Build history of the part. All positions in model axes, mm. A direction names the side the tool comes from. Coordinates: 2 decimals unless noted, no trailing zeros. Write each loop counter-clockwise with the first axis right and the second up, starting at its lowest first coordinate (ties: lowest second). Pieces come first, ordered by that corner, then holes.
Autodesk Inventor part; units mm, degrees
ref_plane "YZ Plane" through (0, 0, 0) normal (1, 0, 0) x (0, 1, 0)
ref_plane "XZ Plane" through (0, 0, 0) normal (0, 1, 0) x (-1, 0, 0)
ref_plane "XY Plane" through (0, 0, 0) normal (0, 0, 1) x (1, 0, 0)
sketch "Sketch1" plane through (0, 0, 0) normal (0, 1, 0) x (-1, 0, 0)
  circle A0 centre (0, 0) radius 4
  dimension "d0" = 8
extrude "Extrusion1" add sketch "Sketch1" along normal blind 9.3
sketch "Sketch2" plane through (0, 9.3, 0) normal (0, 1, 0) x (1, 0, 0)
  line L0 (2.8284, 2.8284) -> (-2.8284, 2.8284)
  line L1 (-2.8284, 2.8284) -> (-2.8284, -2.8284)
  line L2 (-2.8284, -2.8284) -> (2.8284, -2.8284)
  line L3 (2.8284, -2.8284) -> (2.8284, 2.8284)
  line L4 (2.8284, 2.8284) -> (-2.8284, -2.8284) construction
  line L5 (-2.8284, 2.8284) -> (2.8284, -2.8284) construction
  circle A0 centre (0, 0) radius 4
extrude "Extrusion2" add sketch "Sketch2" along normal blind 22 contours L3 L2 L1 L0
sketch "Sketch3" plane through (0, 0, 0) normal (0, -1, 0) x (1, 0, 0)
  line L0 (2.8284, -2.8284) -> (-2.8284, -2.8284)
  line L1 (-2.8284, -2.8284) -> (-2.8284, 2.8284)
  line L2 (-2.8284, 2.8284) -> (2.8284, 2.8284)
  line L3 (2.8284, 2.8284) -> (2.8284, -2.8284)
  line L4 (2.8284, -2.8284) -> (-2.8284, 2.8284) construction
  line L5 (-2.8284, -2.8284) -> (2.8284, 2.8284) construction
  circle A0 centre (0, 0) radius 4
extrude "Extrusion3" add sketch "Sketch3" along normal blind 15.7 contours L0 L1 L2 L3
properties part number "SCARA swivel connection rod"
1. Saw through at C-C on y = -2. List the corners of the cut face in (x, z).
Computed values:
outline: (-2.83, -2.83) - (2.83, -2.83) - (2.83, 2.83) - (-2.83, 2.83) - close
2. Saw through at B-B on x = 0. List the corners of the cut face in (y, z), plus the area to 3 significant figures.
Computed values:
outline: (-15.7, -2.83) - (0, -2.83) - (0, -4) - (9.3, -4) - (9.3, -2.83) - (31.3, -2.83) - (31.3, 2.83) - (9.3, 2.83) - (9.3, 4) - (0, 4) - (0, 2.83) - (-15.7, 2.83) - close
area: 288 mm2
3. Flat gauge pins, fed straight in: pin 1 (4.5 mm diameter, centred on x = -0.5, y = 22.5, fed in from -Z); pin 2 (3 mm diameter, centred on y = -5, z = -0.5, fed in from +X); pin 3 (4.5 mm diameter, centred on y = -7.5, z = 1, fed in from -X). Where does each tip first touch, or does it go through?
Computed values:
pin 1: stops at z = -2.83
pin 2: stops at x = 2.83
pin 3: stops at x = -2.83
4. Saw through at A-A on z = 0. List the corners of the cut face in (x, y), plus the area to 3 significant figures.
Computed values:
outline: (-4, 0) - (-2.83, 0) - (-2.83, -15.7) - (2.83, -15.7) - (2.83, 0) - (4, 0) - (4, 9.3) - (2.83, 9.3) - (2.83, 31.3) - (-2.83, 31.3) - (-2.83, 9.3) - (-4, 9.3) - close
area: 288 mm2
5. Probe line 1 along Z through (x, y) = (1, 21.5); line 2 along Z through (x, y) = (3.25, 9). List the from-to ranges inside material, lowest first.
Computed values:
line 1: z = -2.83 to 2.83
line 2: z = -2.33 to 2.33
6. 3-axis set-ups, long thin cutter, end or side, ignore diameter. For faces 1 (the face through (-3, 0, 0)), 2 (the face through (-3, 9.3, 0)), 3 (the face through (0, 20, -2.828)), 4 (the face through (0, 0, 3)), 5 (the face through (0, 9.3, 3)): which of +Z, -Z, +X, -X, +Y, -Y reach the whole face in a straight line?
Computed values:
face 1: +Z, -Z, -X, -Y
face 2: +Z, -Z, -X, +Y
face 3: -Z, +X, -X, +Y
face 4: +Z, +X, -X, -Y
face 5: +Z, +X, -X, +Y
